The figure shows three views and two pictorial views of one solid part (mm, origin at its lowest corner). Answer the questions. A direction names the side the tool comes from. Round coordinates to 2 decimals unless told otherwise and drop trailing zeros. Loops run counter-clockwise (first coordinate to the right, second up) from the corner with the lowest first, then second, coordinate; pieces in that order, holes last. Notation, with made-up numbers: (84.5, 58.25) -> (119.5, 58.25) arc R22 ccw to (119.5, 65.25) -> close; hole circle Ø10 at (53.5, 72). An arc over 180 degrees is marked (long way). Use a Markdown table: item, result. Add a question column.
Q1. Section C-C on x = 13.2 is taken. Give the vertices of the cut face in (y, z).
Q2. Consider line 1 (X direction, y = 3.75, z = 26); line 2 (Z direction, x = 13.2, y = 8.5); line 3 (Z direction, x = 11.5, y = 2). Determine where each line is inside the solid, lowest interval first.
Q3. Section B-B on y = 4.5 is taken. Give the vertices of the cut face in (x, z), then the cut area to 3 significant figures.
Q4. Section A-A on z = 26 is taken. Give the vertices of the cut face in (x, y).
Q5. Section D-D on x = 19 is taken. Give the vertices of the cut face in (y, z), then the cut area to 3 significant figures.
Q6. Which of the six approach directions +Z, -Z, +X, -X, +Y, -Y give full straight-line access (tool end or side, diameter ignored) to the marked faces 1, 2 and 3?
Q7. Given pin 1 Ø3 at (x, y) = (15, 8) entering from +Z; pin 2 Ø3 at (y, z) = (5.5, 36) entering from +X; pin 3 Ø6.5 at (x, z) = (9, 3) entering from -Y, each flat-ended and moving along its own axis, determine where each tip first touches the part or whether it passes through.
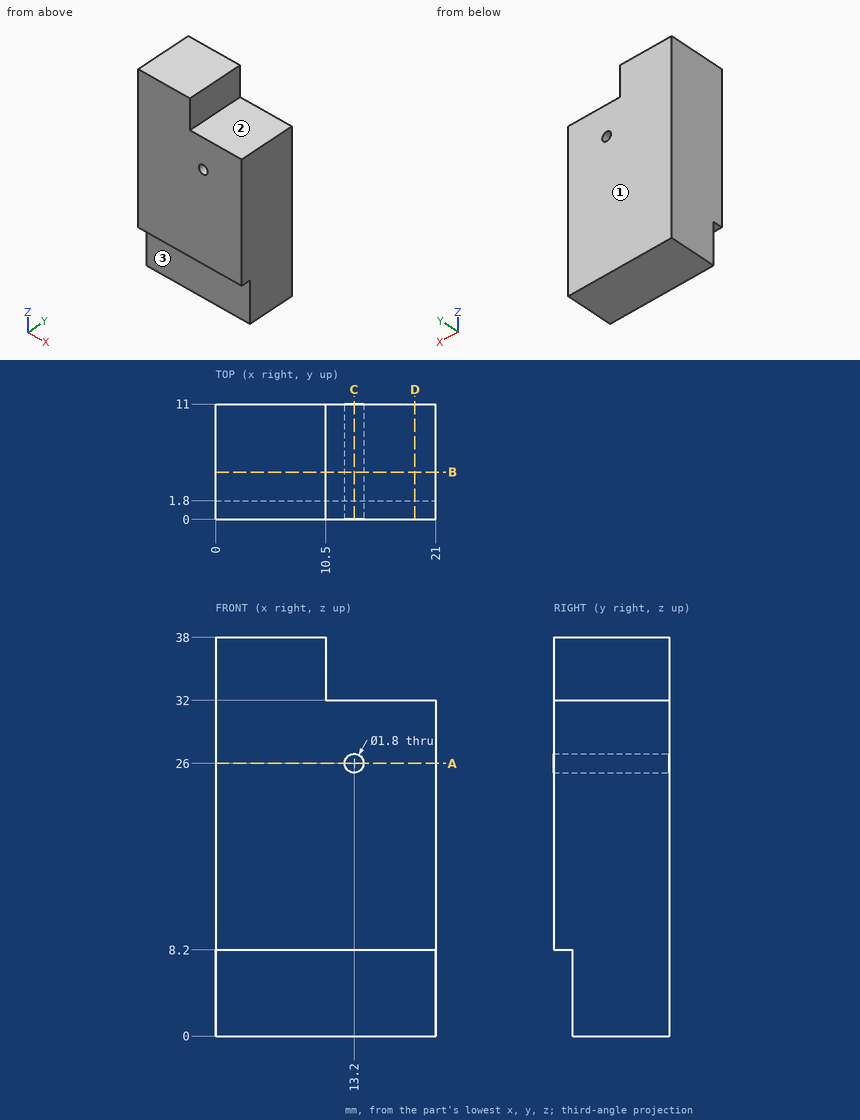
Checked values:
| question | item | result |
|---|---|---|
| 1 | outline | (0, 8.2) -> (1.8, 8.2) -> (1.8, 0) -> (11, 0) -> (11, 25.1) -> (0, 25.1) -> close; (0, 26.9) -> (11, 26.9) -> (11, 32) -> (0, 32) -> close |
| 2 | line 1 | x = 0 to 12.3, 14.1 to 21 |
| 2 | line 2 | z = 0 to 25.1, 26.9 to 32 |
| 2 | line 3 | z = 0 to 32 |
| 3 | outline | (0, 0) -> (21, 0) -> (21, 32) -> (10.5, 32) -> (10.5, 38) -> (0, 38) -> close; hole circle Ø1.8 at (13.2, 26) |
| 3 | area | 732 mm2 |
| 4 | outline | (0, 0) -> (12.3, 0) -> (12.3, 11) -> (0, 11) -> close; (14.1, 0) -> (21, 0) -> (21, 11) -> (14.1, 11) -> close |
| 5 | outline | (0, 8.2) -> (1.8, 8.2) -> (1.8, 0) -> (11, 0) -> (11, 32) -> (0, 32) -> close |
| 5 | area | 337 mm2 |
| 6 | face 1 | +Z, -Z, +X, -X, +Y |
| 6 | face 2 | +Z, +X, +Y, -Y |
| 6 | face 3 | -Z, +X, -X, -Y |
| 7 | pin 1 | stops at z = 32 |
| 7 | pin 2 | stops at x = 10.5 |
| 7 | pin 3 | stops at y = 1.8 |
